```python
from build123d import *

# Parameters (mm, degrees)
SKETCH1_R           = 19.54
SKETCH1_R_2         = 15.54
BOSS_EXTRUDE1_DEPTH = 7.9
SKETCH1_3_R         = 2.7
BOSS_EXTRUDE2_DEPTH = 7.9
SKETCH1_4_R         = 1.5
CUT_EXTRUDE1_DEPTH  = 29.740793308
CUT_EXTRUDE2_DEPTH  = 29.740793308
SKETCH1_6_R         = 1.5
CUT_EXTRUDE5_DEPTH  = 3
CIRPATTERN1_COUNT   = 3
SKETCH2_R           = 26
SKETCH2_R_2         = 19.54
BOSS_EXTRUDE3_DEPTH = 7.9
CUT_EXTRUDE4_START  = 7.9
SKETCH2_3_R         = 22
SKETCH2_3_R_2       = 19.54
CUT_EXTRUDE4_DEPTH  = 3.14
CUT_EXTRUDE6_START  = 3
SKETCH2_4_R         = 22
CUT_EXTRUDE6_DEPTH  = 3


with BuildPart() as part:
    # Sketch1 → Boss-Extrude1 (new body)
    with BuildSketch(Plane(origin=(0, 0, 0), x_dir=(1, 0, 0), z_dir=(0, 1, 0))):
        with Locations(Location((0, 0, 0), (0, 0, 270))):
            Circle(SKETCH1_R)
        with Locations(Location((0, 0, 0), (0, 0, 270))):
            Circle(SKETCH1_R_2, mode=Mode.SUBTRACT)
    extrude(amount=BOSS_EXTRUDE1_DEPTH)

    # Sketch1<3> → Boss-Extrude2 (add)
    with BuildSketch(Plane(origin=(0, 0, 0), x_dir=(1, 0, 0), z_dir=(0, 1, 0))):
        with Locations((15.54, 0)):
            Circle(SKETCH1_3_R)
    boss_extrude2 = extrude(amount=BOSS_EXTRUDE2_DEPTH)

    # Sketch1<4> → Cut-Extrude1 (cut, symmetric)
    with BuildSketch(Plane(origin=(0, 0, 0), x_dir=(1, 0, 0), z_dir=(0, 1, 0))):
        with Locations(Location((15.54, 0, 0), (0, 0, 270))):
            Circle(SKETCH1_4_R)
    cut_extrude1 = extrude(amount=CUT_EXTRUDE1_DEPTH, both=True, mode=Mode.SUBTRACT)

    # Sketch1<5> → Cut-Extrude2 (cut, symmetric)
    with BuildSketch(Plane(origin=(0, 0, 0), x_dir=(1, 0, 0), z_dir=(0, 1, 0))):
        with BuildLine():
            Line((1.84893352, 16.641004923), (1.716044464, 15.444960065))
            ThreePointArc((1.716044464, 15.444960065), (7.546281877, 13.584742538), (12.206193142, 9.617715372))
            Line((12.206193142, 9.617715372), (13.151430585, 10.362503249))
            ThreePointArc((13.151430585, 10.362503249), (13.623726964, 11.24345363), (13.299320972, 12.188915525))
            ThreePointArc((13.299320972, 12.188915525), (8.760291222, 15.770190161), (3.321432407, 17.731601359))
            ThreePointArc((3.321432407, 17.731601359), (2.347317501, 17.507463762), (1.84893352, 16.641004923))
        make_face()
    cut_extrude2 = extrude(amount=CUT_EXTRUDE2_DEPTH, both=True, mode=Mode.SUBTRACT)

    # Sketch1<6> → Cut-Extrude5 (cut)
    with BuildSketch(Plane(origin=(0, 0, 0), x_dir=(1, 0, 0), z_dir=(0, 1, 0))):
        with BuildLine():
            Line((13.541549805, -7.623518144), (14.590196156, -8.213877046))
            ThreePointArc((14.590196156, -8.213877046), (15.584628409, -8.315079224), (16.335293585, -7.655049543))
            ThreePointArc((16.335293585, -7.655049543), (17.48108114, -4.455715676), (18.006537967, -1.098267026))
            ThreePointArc((18.006537967, -1.098267026), (18.24, 0), (18.006537967, 1.098267026))
            ThreePointArc((18.006537967, 1.098267026), (17.48108114, 4.455715676), (16.335293585, 7.655049543))
            ThreePointArc((16.335293585, 7.655049543), (15.584628409, 8.315079224), (14.590196156, 8.213877046))
            Line((14.590196156, 8.213877046), (13.541549805, 7.623518144))
            ThreePointArc((13.541549805, 7.623518144), (14.632931196, 5.231531765), (15.305444015, 2.689792462))
            ThreePointArc((15.305444015, 2.689792462), (12.84, 0), (15.305444015, -2.689792462))
            ThreePointArc((15.305444015, -2.689792462), (14.632931196, -5.231531765), (13.541549805, -7.623518144))
        make_face()
        with Locations(Location((15.54, 0, 0), (0, 0, 270))):
            Circle(SKETCH1_6_R, mode=Mode.SUBTRACT)
    cut_extrude5 = extrude(amount=CUT_EXTRUDE5_DEPTH, mode=Mode.SUBTRACT)

    # CirPattern1: Boss-Extrude2, Cut-Extrude1, Cut-Extrude2, Cut-Extrude5 ×3 about axis
    cirpattern1_axis = Axis((0, 0, 0), (0, 1, 0))
    add([boss_extrude2.rotate(cirpattern1_axis, i * 360 / CIRPATTERN1_COUNT) for i in range(1, CIRPATTERN1_COUNT)])
    add([cut_extrude1.rotate(cirpattern1_axis, i * 360 / CIRPATTERN1_COUNT) for i in range(1, CIRPATTERN1_COUNT)], mode=Mode.SUBTRACT)
    add([cut_extrude2.rotate(cirpattern1_axis, i * 360 / CIRPATTERN1_COUNT) for i in range(1, CIRPATTERN1_COUNT)], mode=Mode.SUBTRACT)
    add([cut_extrude5.rotate(cirpattern1_axis, i * 360 / CIRPATTERN1_COUNT) for i in range(1, CIRPATTERN1_COUNT)], mode=Mode.SUBTRACT)

    # Sketch2 → Boss-Extrude3 (add)
    with BuildSketch(Plane(origin=(0, 0, 0), x_dir=(1, 0, 0), z_dir=(0, 1, 0))):
        with Locations(Location((0, 0, 0), (0, 0, 270))):
            Circle(SKETCH2_R)
        Circle(SKETCH2_R_2, mode=Mode.SUBTRACT)
    extrude(amount=BOSS_EXTRUDE3_DEPTH)

    # Sketch2<3> → Cut-Extrude4 (cut)
    with BuildSketch(Plane(origin=(0, 0, 0), x_dir=(1, 0, 0), z_dir=(0, 1, 0)).offset(CUT_EXTRUDE4_START)):
        with Locations(Location((0, 0, 0), (0, 0, 270))):
            Circle(SKETCH2_3_R)
        with Locations(Location((0, 0, 0), (0, 0, 270))):
            Circle(SKETCH2_3_R_2, mode=Mode.SUBTRACT)
    extrude(amount=-CUT_EXTRUDE4_DEPTH, mode=Mode.SUBTRACT)

    # Sketch2<4> → Cut-Extrude6 (cut)
    with BuildSketch(Plane(origin=(0, 0, 0), x_dir=(1, 0, 0), z_dir=(0, 1, 0)).offset(CUT_EXTRUDE6_START)):
        with Locations(Location((0, 0, 0), (0, 0, 270))):
            Circle(SKETCH2_4_R)
    extrude(amount=-CUT_EXTRUDE6_DEPTH, mode=Mode.SUBTRACT)


solid = part.part
```
Verification items for the finished model (mm, model axes). A direction names the side the tool comes from. Round coordinates to 2 decimals unless told otherwise and drop trailing zeros. Write each loop counter-clockwise with the first axis right and the second up, starting at its lowest first coordinate (ties: lowest second). Pieces come first, ordered by that corner, then holes.
1. Section check B-B on x = -12. Enter the section's corners in (y, z), plus the area to 3 significant figures.
2. Access from +Z, -Z, +X, -X, +Y, -Y to the whole of each face (thin tool, end or side, straight path). Record for faces 4 (the cylindrical face through (14.269, 5.416, 6.156)), 5 (the flat face through (-5, 3, -15)).
3. Gauge pin test, flat ends, axial feed: P1, Ø2, axis at y = 5.5, z = 2.5, coming from the +X side; P2, Ø22, axis at x = 2, z = 10, coming from the -Y side; P3, Ø1.5, axis at x = 8, y = 3.5, coming from the +Z side; P4, Ø5, axis at x = -7.77, z = 13.46, coming from the +Y side. Record the tip position at first contact, or that the pin passes through.
4. Section check D-D on z = 13.5. Enter the section's corners in (x, y).
5. Section check C-C on y = 1. Enter the section's corners in (x, z).
6. Section check A-A on z = 0. Enter the section's corners in (x, y).
7. Scan lines: L1, parallel to X at y = 7.75, z = 7.5; L2, parallel to X at y = 4.05, z = 0; L3, parallel to X at y = 6.75, z = -14.5. Record each from-to range of solid material in increasing order.
8. Draft check along Z on faces 1 (the flat face through (13, 7.9, 0)), 2 (the cylindrical face through (-15.821, 3.895, -20.633)), 3 (the cylindrical face through (12.84, 5.42, -0.06)). Enter one of: +Z half, -Z half, draft (parallel to the pull), parting line (faces both ways), or undercut.
Answer:
1. outline: (0, -23.07) - (7.9, -23.07) - (7.9, -18.44) - (4.76, -18.44) - (4.76, -15.42) - (7.9, -15.42) - (7.9, -9.87) - (3, -9.87) - (3, -18.44) - (0, -18.44) - close; (0, 18.44) - (3, 18.44) - (3, 9.87) - (7.9, 9.87) - (7.9, 15.42) - (4.76, 15.42) - (4.76, 18.44) - (7.9, 18.44) - (7.9, 23.07) - (0, 23.07) - close
1. area: 138 mm2
2. face 4: +Y, -Y
2. face 5: -Y
3. P1: stops at x = 25.96
3. P2: stops at y = 3
3. P3: stops at z = 24.97
3. P4: stops at y = 7.9
4. outline: (-22.22, 0) - (-17.37, 0) - (-17.37, 3) - (-9.27, 3) - (-9.27, 7.9) - (-14.13, 7.9) - (-14.13, 4.76) - (-17.37, 4.76) - (-17.37, 7.9) - (-22.22, 7.9) - close; (-6.27, 3) - (-5.07, 3) - (-5.07, 7.9) - (-6.27, 7.9) - close; (11.97, 3) - (17.37, 3) - (17.37, 0) - (22.22, 0) - (22.22, 7.9) - (17.37, 7.9) - (17.37, 4.76) - (14.13, 4.76) - (14.13, 7.9) - (11.97, 7.9) - close
5. outline: circle Ø52 at (0, 0); hole circle Ø44 at (0, 0)
6. outline: (-26, 0) - (-22, 0) - (-22, 3) - (-18.04, 3) - (-18.04, 7.9) - (-19.54, 7.9) - (-19.54, 4.76) - (-22, 4.76) - (-22, 7.9) - (-26, 7.9) - close; (12.84, 3) - (14.04, 3) - (14.04, 7.9) - (12.84, 7.9) - close; (17.04, 3) - (22, 3) - (22, 0) - (26, 0) - (26, 7.9) - (22, 7.9) - (22, 4.76) - (19.54, 4.76) - (19.54, 7.9) - (17.04, 7.9) - close
7. L1: x = -24.89 to -20.68, -18.04 to -13.61, 13.61 to 18.04, 20.68 to 24.89
7. L2: x = -26 to -18.04, 12.84 to 14.04, 17.04 to 26
7. L3: x = -21.58 to -16.55, -13.1 to -8.85, -6.69 to -5.28, 10.73 to 13.1, 16.55 to 21.58
8. face 1: draft
8. face 2: parting line
8. face 3: undercut
